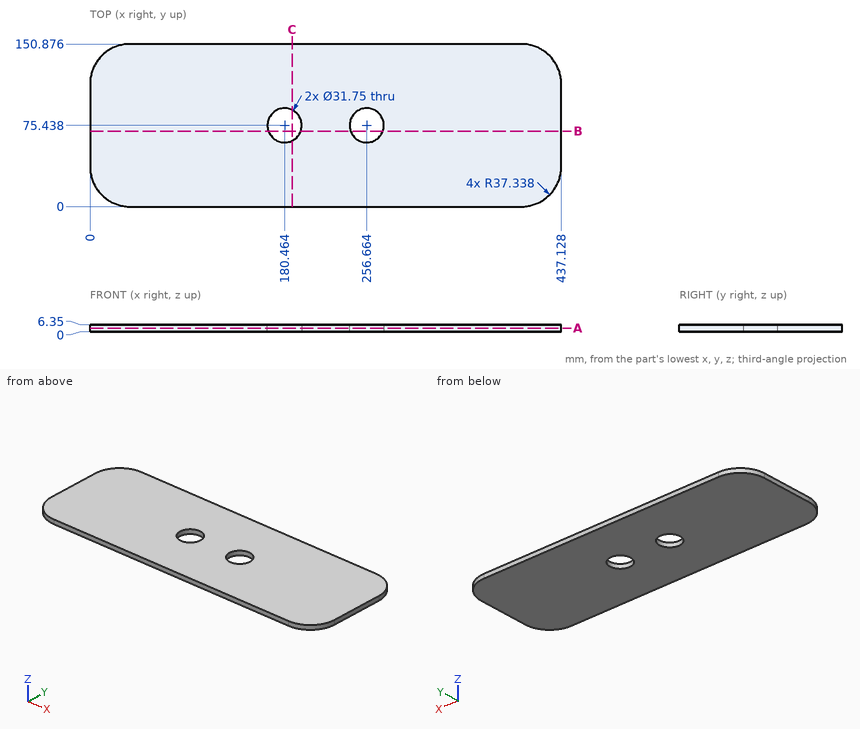
Design review of the part shown in the three views and the two pictorial views. Dimensions are in mm from the part's minimum x, y and z. Round coordinates to 2 decimals unless told otherwise and drop trailing zeros. Order: outer loops, then holes, each group sorted by start corner. A loop starts at its lowest first (then second) coordinate and runs counter-clockwise, first axis right, second up.
(1) Take a section at C-C, the plane x = 187.5. State the section outline as (y, z) points.
Working result:
outline: (0, 0) - (61.21, 0) - (61.21, 6.35) - (0, 6.35) - close; (89.67, 0) - (150.88, 0) - (150.88, 6.35) - (89.67, 6.35) - close
(2) Take a section at B-B, the plane y = 70. State the section outline as (x, z) points.
Working result:
outline: (0, 0) - (165.55, 0) - (165.55, 6.35) - (0, 6.35) - close; (195.38, 0) - (241.75, 0) - (241.75, 6.35) - (195.38, 6.35) - close; (271.58, 0) - (437.13, 0) - (437.13, 6.35) - (271.58, 6.35) - close
(3) Take a section at A-A, the plane z = 3.25. Count the separate pieces of the cut face and the enclosed holes in it, plus the area to 3 significant figures.
Working result:
separate pieces: 1
enclosed holes: 2
area: 63,200 mm2
(4) For P1, Ø1, axis at y = 20.5, z = 3, coming from the -X side (1 decimal); P2, Ø3, axis at y = 120.5, z = 5.5, coming from the -X side, all flat-tipped, find the tip position at first contact; note any pin that passes through.
Working result:
P1: stops at x = 3.8
P2: stops at x = 0.4
(5) Wall thickness on L1, parallel to X at y = 66, z = 1; L2, parallel to X at y = 68, z = 2.75; L3, parallel to X at y = 114, z = 0.5 (1 decimal): over which ranges is each line inside the solid? List them lowest first.
Working result:
L1: x = 0 to 167.7, 193.23 to 243.9, 269.43 to 437.13
L2: x = 0 to 166.44, 194.49 to 242.64, 270.69 to 437.13
L3: x = 0 to 437.1
